```python
from build123d import *

# Parameters (mm, degrees)
SKETCH_1_R      = 2.25
SKETCH_1_R_2    = 1.5
SKETCH_1_W      = 5
SKETCH_1_H      = 20
SKETCH_1_W_2    = 20
SKETCH_1_H_2    = 5
EXTRUDE_1_DEPTH = 5


with BuildPart() as part:
    # 草图1 → 凸台-拉伸1 (new body)
    with BuildSketch(Plane(origin=(0, 0, 0), x_dir=(0, 0, -1), z_dir=(1, 0, 0))):
        with BuildLine():
            Line((-168.536416178, -19.716908756), (-168.536416178, -16.716908756))
            ThreePointArc((-168.536416178, -16.716908756), (-167.950629741, -15.302695194), (-166.536416178, -14.716908756))
            Line((-166.536416178, -14.716908756), (69.463583822, -14.716908756))
            ThreePointArc((69.463583822, -14.716908756), (70.877797384, -15.302695194), (71.463583822, -16.716908756))
            Line((71.463583822, -16.716908756), (71.463583822, -19.716908756))
            ThreePointArc((71.463583822, -19.716908756), (72.928049916, -23.252442662), (76.463583822, -24.716908756))
            Line((76.463583822, -24.716908756), (116.463583822, -24.716908756))
            ThreePointArc((116.463583822, -24.716908756), (119.999117728, -23.252442662), (121.463583822, -19.716908756))
            Line((121.463583822, -19.716908756), (121.463583822, 12.583091244))
            Line((121.463583822, 12.583091244), (126.463583822, 12.583091244))
            Line((126.463583822, 12.583091244), (126.463583822, 32.583091244))
            Line((126.463583822, 32.583091244), (121.463583822, 32.583091244))
            Line((121.463583822, 32.583091244), (121.463583822, 41.083091244))
            Line((121.463583822, 41.083091244), (118.463583822, 41.083091244))
            Line((118.463583822, 41.083091244), (118.463583822, 39.833091244))
            Line((118.463583822, 39.833091244), (115.463583822, 39.833091244))
            Line((115.463583822, 39.833091244), (115.463583822, 41.083091244))
            Line((115.463583822, 41.083091244), (113.463583822, 41.083091244))
            Line((113.463583822, 41.083091244), (113.463583822, 44.083091244))
            Line((113.463583822, 44.083091244), (115.463583822, 44.083091244))
            Line((115.463583822, 44.083091244), (115.463583822, 45.333091244))
            Line((115.463583822, 45.333091244), (118.463583822, 45.333091244))
            Line((118.463583822, 45.333091244), (118.463583822, 44.083091244))
            Line((118.463583822, 44.083091244), (121.463583822, 44.083091244))
            Line((121.463583822, 44.083091244), (121.463583822, 52.583091244))
            Line((121.463583822, 52.583091244), (126.463583822, 52.583091244))
            Line((126.463583822, 52.583091244), (126.463583822, 72.583091244))
            Line((126.463583822, 72.583091244), (121.463583822, 72.583091244))
            Line((121.463583822, 72.583091244), (121.463583822, 81.083091244))
            Line((121.463583822, 81.083091244), (118.463583822, 81.083091244))
            Line((118.463583822, 81.083091244), (118.463583822, 79.833091244))
            Line((118.463583822, 79.833091244), (115.463583822, 79.833091244))
            Line((115.463583822, 79.833091244), (115.463583822, 81.083091244))
            Line((115.463583822, 81.083091244), (113.463583822, 81.083091244))
            Line((113.463583822, 81.083091244), (113.463583822, 84.083091244))
            Line((113.463583822, 84.083091244), (115.463583822, 84.083091244))
            Line((115.463583822, 84.083091244), (115.463583822, 85.333091244))
            Line((115.463583822, 85.333091244), (118.463583822, 85.333091244))
            Line((118.463583822, 85.333091244), (118.463583822, 84.083091244))
            Line((118.463583822, 84.083091244), (121.463583822, 84.083091244))
            Line((121.463583822, 84.083091244), (121.463583822, 92.583091244))
            Line((121.463583822, 92.583091244), (-218.536416178, 92.583091244))
            Line((-218.536416178, 92.583091244), (-218.536416178, 84.083091244))
            Line((-218.536416178, 84.083091244), (-215.536416178, 84.083091244))
            Line((-215.536416178, 84.083091244), (-215.536416178, 85.333091244))
            Line((-215.536416178, 85.333091244), (-212.536416178, 85.333091244))
            Line((-212.536416178, 85.333091244), (-212.536416178, 84.083091244))
            Line((-212.536416178, 84.083091244), (-210.536416178, 84.083091244))
            Line((-210.536416178, 84.083091244), (-210.536416178, 81.083091244))
            Line((-210.536416178, 81.083091244), (-212.536416178, 81.083091244))
            Line((-212.536416178, 81.083091244), (-212.536416178, 79.833091244))
            Line((-212.536416178, 79.833091244), (-215.536416178, 79.833091244))
            Line((-215.536416178, 79.833091244), (-215.536416178, 81.083091244))
            Line((-215.536416178, 81.083091244), (-218.536416178, 81.083091244))
            Line((-218.536416178, 81.083091244), (-218.536416178, 72.583091244))
            Line((-218.536416178, 72.583091244), (-223.536416178, 72.583091244))
            Line((-223.536416178, 72.583091244), (-223.536416178, 52.583091244))
            Line((-223.536416178, 52.583091244), (-218.536416178, 52.583091244))
            Line((-218.536416178, 52.583091244), (-218.536416178, 44.083091244))
            Line((-218.536416178, 44.083091244), (-215.536416178, 44.083091244))
            Line((-215.536416178, 44.083091244), (-215.536416178, 45.333091244))
            Line((-215.536416178, 45.333091244), (-212.536416178, 45.333091244))
            Line((-212.536416178, 45.333091244), (-212.536416178, 44.083091244))
            Line((-212.536416178, 44.083091244), (-210.536416178, 44.083091244))
            Line((-210.536416178, 44.083091244), (-210.536416178, 41.083091244))
            Line((-210.536416178, 41.083091244), (-212.536416178, 41.083091244))
            Line((-212.536416178, 41.083091244), (-212.536416178, 39.833091244))
            Line((-212.536416178, 39.833091244), (-215.536416178, 39.833091244))
            Line((-215.536416178, 39.833091244), (-215.536416178, 41.083091244))
            Line((-215.536416178, 41.083091244), (-218.536416178, 41.083091244))
            Line((-218.536416178, 41.083091244), (-218.536416178, 32.583091244))
            Line((-218.536416178, 32.583091244), (-223.536416178, 32.583091244))
            Line((-223.536416178, 32.583091244), (-223.536416178, 12.583091244))
            Line((-223.536416178, 12.583091244), (-218.536416178, 12.583091244))
            Line((-218.536416178, 12.583091244), (-218.536416178, -19.716908756))
            ThreePointArc((-218.536416178, -19.716908756), (-217.071950084, -23.252442662), (-213.536416178, -24.716908756))
            Line((-213.536416178, -24.716908756), (-173.536416178, -24.716908756))
            ThreePointArc((-173.536416178, -24.716908756), (-170.000882272, -23.252442662), (-168.536416178, -19.716908756))
        make_face()
        with Locations((27.463583822, 34.283091244)):
            Circle(SKETCH_1_R, mode=Mode.SUBTRACT)
        with Locations((-12.536416178, 34.283091244)):
            Circle(SKETCH_1_R, mode=Mode.SUBTRACT)
        with Locations((-38.036416178, 42.583091244)):
            Circle(SKETCH_1_R_2, mode=Mode.SUBTRACT)
        with Locations((-158.036416178, 42.583091244)):
            Circle(SKETCH_1_R_2, mode=Mode.SUBTRACT)
        with Locations((-38.036416178, 62.583091244)):
            Rectangle(SKETCH_1_W, SKETCH_1_H, mode=Mode.SUBTRACT)
        with Locations((-38.036416178, 22.583091244)):
            Rectangle(SKETCH_1_W, SKETCH_1_H, mode=Mode.SUBTRACT)
        with Locations((-158.036416178, 62.583091244)):
            Rectangle(SKETCH_1_W, SKETCH_1_H, mode=Mode.SUBTRACT)
        with Locations((-158.036416178, 22.583091244)):
            Rectangle(SKETCH_1_W, SKETCH_1_H, mode=Mode.SUBTRACT)
        with Locations((-118.536416178, -7.216908756)):
            Rectangle(SKETCH_1_W_2, SKETCH_1_H_2, mode=Mode.SUBTRACT)
        with Locations((-188.536416178, -7.216908756)):
            Rectangle(SKETCH_1_W_2, SKETCH_1_H_2, mode=Mode.SUBTRACT)
        with Locations((101.463583822, -7.216908756)):
            Rectangle(SKETCH_1_W_2, SKETCH_1_H_2, mode=Mode.SUBTRACT)
        with Locations((51.463583822, -7.216908756)):
            Rectangle(SKETCH_1_W_2, SKETCH_1_H_2, mode=Mode.SUBTRACT)
        with BuildLine():
            Line((18.463583822, 58.283091244), (-3.536416178, 58.283091244))
            ThreePointArc((-3.536416178, 58.283091244), (-5.657736522, 57.404411587), (-6.536416178, 55.283091244))
            Line((-6.536416178, 55.283091244), (-6.536416178, 13.283091244))
            ThreePointArc((-6.536416178, 13.283091244), (-5.657736522, 11.1617709), (-3.536416178, 10.283091244))
            Line((-3.536416178, 10.283091244), (18.463583822, 10.283091244))
            ThreePointArc((18.463583822, 10.283091244), (20.584904165, 11.1617709), (21.463583822, 13.283091244))
            Line((21.463583822, 13.283091244), (21.463583822, 55.283091244))
            ThreePointArc((21.463583822, 55.283091244), (20.584904165, 57.404411587), (18.463583822, 58.283091244))
        make_face(mode=Mode.SUBTRACT)
        with BuildLine():
            Line((-125.536416178, 57.583091244), (-96.536416178, 57.583091244))
            ThreePointArc((-96.536416178, 57.583091244), (-94.415095835, 56.704411587), (-93.536416178, 54.583091244))
            Line((-93.536416178, 54.583091244), (-93.536416178, 50.583091244))
            ThreePointArc((-93.536416178, 50.583091244), (-94.415095835, 48.4617709), (-96.536416178, 47.583091244))
            Line((-96.536416178, 47.583091244), (-125.536416178, 47.583091244))
            ThreePointArc((-125.536416178, 47.583091244), (-127.657736522, 48.4617709), (-128.536416178, 50.583091244))
            Line((-128.536416178, 50.583091244), (-128.536416178, 54.583091244))
            ThreePointArc((-128.536416178, 54.583091244), (-127.657736522, 56.704411587), (-125.536416178, 57.583091244))
        make_face(mode=Mode.SUBTRACT)
    extrude(amount=EXTRUDE_1_DEPTH)


solid = part.part
```
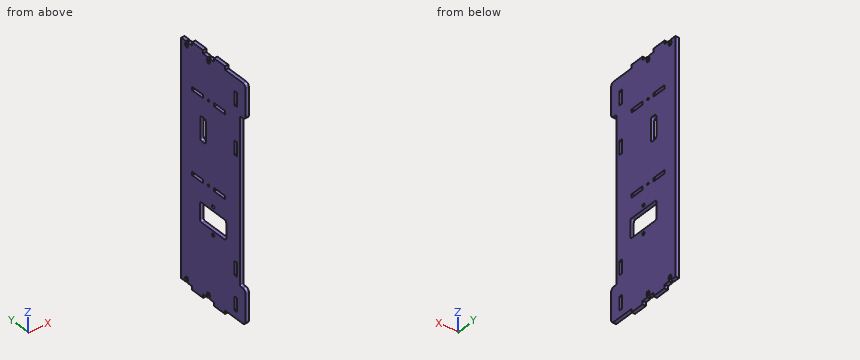
The model under review builds one solid part; all positions refer to its coordinate system, in mm. Give positions to 0.01 mm unless a question says otherwise; leave off trailing zeros. Loops run counter-clockwise (first coordinate to the right, second up) from the corner with the lowest first, then second, coordinate; pieces in that order, holes last. Notation, with made-up numbers: (47.25, 39.25) - (82.25, 39.25) arc R23 ccw to (82.25, 49.25) - close; hole circle Ø11 at (49, 14.5). An arc over 180 degrees is marked (long way). Answer as a JSON object with one key per item and string values.
Q1. Add section A-A on y = 25. State the section outline as (x, z) points, plus the area to 3 significant figures.
Worked out:
{"outline": "(0, -126.46) - (5, -126.46) - (5, -21.46) - (0, -21.46) - close; (0, 6.54) - (5, 6.54) - (5, 35.54) - (0, 35.54) - close; (0, 40.54) - (5, 40.54) - (5, 155.54) - (0, 155.54) - close; (0, 160.54) - (5, 160.54) - (5, 223.54) - (0, 223.54) - close", "area": "1,560 mm^2"}
Q2. Add section D-D on y = 3. State the section outline as (x, z) points, plus the area to 3 significant figures.
Worked out:
{"outline": "(0, -121.46) - (5, -121.46) - (5, 218.54) - (0, 218.54) - close", "area": "1,700 mm^2"}
Q3. Insertion check: pin 1 (1.5 mm diameter, centred on x = 4.5, z = -9, fed in from -Y); pin 2 (3 mm diameter, centred on x = 1.5, z = 165.5, fed in from -Y); pin 3 (0.9 mm diameter, centred on x = 3.5, z = 214, fed in from -Y); pin 4 (2.5 mm diameter, centred on x = 1.5, y = 89, fed in from +Z). Each pin has a flat end and moves straight along its axis. Give the tip position at first contact, or say it passes through.
Worked out:
{"pin 1": "stops at y = -14.72", "pin 2": "stops at y = -14.77", "pin 3": "stops at y = -24.72", "pin 4": "stops at z = 218.54"}
Q4. Add section C-C on y = 66. State the section outline as (x, z) points.
Worked out:
{"outline": "(0, -126.46) - (5, -126.46) - (5, 35.54) - (0, 35.54) - close; (0, 40.54) - (5, 40.54) - (5, 155.54) - (0, 155.54) - close; (0, 160.54) - (5, 160.54) - (5, 223.54) - (0, 223.54) - close"}
Q5. To check wall thickness, follow line 1 along Z through (x, y) = (4.05, 66.5); line 2 along Z through (x, y) = (1.1, 16.5); line 3 along Y through (x, z) = (1.35, -16.5). State the ranges of each line that lie inside material, in increasing order.
Worked out:
{"line 1": "z = -126.46 to 35.54, 40.54 to 155.54, 160.54 to 223.54", "line 2": "z = -126.46 to -21.46, 6.54 to 35.54, 40.54 to 155.54, 160.54 to 223.54", "line 3": "y = -14.72 to 10.28, 58.28 to 92.58"}
Q6. Add section B-B on z = -98.5. State the section outline as (x, y) points, plus the area to 4 significant figures.
Worked out:
{"outline": "(0, -24.72) - (5, -24.72) - (5, -9.72) - (0, -9.72) - close; (0, -4.72) - (5, -4.72) - (5, 92.58) - (0, 92.58) - close", "area": "561.5 mm^2"}
